For this review, take the finished solid that the model builds, in its own axes (mm). Coordinates: 2 decimals unless noted, no trailing zeros. Loops run counter-clockwise (first coordinate to the right, second up) from the corner with the lowest first, then second, coordinate; pieces in that order, holes last. Notation, with made-up numbers: (55, 64.5) -> (100, 64.5) arc R12 ccw to (100, 71.5) -> close; hole circle Ø7 at (57, -38). An arc over 180 degrees is marked (long way). Use a Markdown table: item, result.
from build123d import *

# Parameters (mm, degrees)
FILLET1_R = 3


with BuildPart() as part:
    # Sketch1 → Revolve1 (revolve)
    with BuildSketch(Plane.XY):
        with BuildLine():
            Line((-15.5, 25), (15.5, 25))
            Line((15.5, 25), (15.5, 37))
            Line((15.5, 37), (8.94427191, 37))
            ThreePointArc((8.94427191, 37), (0, 33), (-8.94427191, 37))
            Line((-8.94427191, 37), (-15.5, 37))
            Line((-15.5, 37), (-15.5, 25))
        make_face()
    revolve(axis=Axis((-22.616352201, 0, 0), (1, 0, 0)))

    # Fillet1
    fillet1_edges = [part.edges().sort_by_distance(p)[0] for p in [
        (15.5, -25, 0),
        (-15.5, -25, 0),
    ]]
    fillet(fillet1_edges, radius=FILLET1_R)


solid = part.part
(1) Take a section at A-A on y = 0. Write out the cut boundary in (x, z).
Found:
| item | result |
|---|---|
| outline | (-15.5, -37) -> (-8.94, -37) arc R12 cw to (8.94, -37) -> (15.5, -37) -> (15.5, -28) arc R3 ccw to (12.5, -25) -> (-12.5, -25) arc R3 ccw to (-15.5, -28) -> close; (-15.5, 28) arc R3 ccw to (-12.5, 25) -> (12.5, 25) arc R3 ccw to (15.5, 28) -> (15.5, 37) -> (8.94, 37) arc R12 cw to (-8.94, 37) -> (-15.5, 37) -> close |
(2) For pin 1 Ø6 at (y, z) = (-29, -28.5) entering from +X; pin 2 Ø5 at (x, y) = (2, -16.5) entering from +Z; pin 3 Ø4 at (x, y) = (-7, -14.5) entering from +Z; pin 4 Ø2 at (x, y) = (-2.5, -5) entering from -Z, all flat-tipped, find the tip position at first contact; note any pin that passes through.
Found:
| item | result |
|---|---|
| pin 1 | passes through |
| pin 2 | stops at z = 30.22 |
| pin 3 | stops at z = 34.25 |
| pin 4 | stops at z = -33.18 |
(3) Take a section at C-C on x = 11.5. Write out the cut boundary in (y, z), plus the area to 3 significant figures.
Found:
| item | result |
|---|---|
| outline | circle Ø74 at (0, 0); hole circle Ø50 at (0, 0) |
| area | 2,340 mm^2 |
(4) Mouldability with a two-part tool opening along Y and no side actions: class faces 1 (the face through (0.175, 23.846, 7.509)), 2 (the face through (-12.27, -8.02, -36.12)), 3 (the face through (15.5, 6, 28)) as pulls with the +Y half, pulls with the -Y half, needs draft (parallel to the pull), parting line crosses it, or undercut.
Found:
| item | result |
|---|---|
| face 1 | undercut |
| face 2 | parting line crosses it |
| face 3 | needs draft |
(5) For line 1 along Y through (x, z) = (6.5, 6); line 2 along Z through (x, y) = (-8, 11); line 3 along Z through (x, y) = (-4.5, 0), list the stretches that pass through material, from the lowest coordinate up.
Found:
| item | result |
|---|---|
| line 1 | y = -34.39 to -24.27, 24.27 to 34.39 |
| line 2 | z = -34.34 to -22.45, 22.45 to 34.34 |
| line 3 | z = -33.88 to -25, 25 to 33.88 |
